Read the model definition and answer for the solid it produces. Units are mm, in the model's axes. A direction names the side the tool comes from. Give positions to 0.01 mm unless a question says otherwise; leave off trailing zeros. Order: outer loops, then holes, each group sorted by start corner. A loop starts at its lowest first (then second) coordinate and runs counter-clockwise, first axis right, second up. Notation, with made-up numbers: (20, 39) -> (49, 39) arc R32 cw to (49, 74) -> close; hole circle Ø8 at (-36, 7). An arc over 180 degrees is marked (long way). Answer as CSV lines item,"result". Start each with the question number.
1) Find section C-C (z = -7). Determine the outline of the cut face in (x, y).
2) Find section B-B (x = -14.5). Determine the outline of the cut face in (y, z), and give its area (3 significant figures).
3) Find section A-A (y = 10). Determine the outline of the cut face in (x, z), and give its area (3 significant figures).
4) Flat-ended cylindrical pins translate along their axes: pin 1 Ø0.9 at (y, z) = (1, -30.5) entering from -X; pin 2 Ø4 at (y, z) = (3.5, -33.5) entering from +X; pin 3 Ø5 at (x, y) = (-10, 8.5) entering from -Z (3 decimals); pin 4 Ø6 at (x, y) = (10, 12) entering from +Z. Find the tip coordinate at first contact, or state that the pin passes through.
5) Straight lines are drawn through the part: L1, parallel to Z at x = -1.5, y = 1; L2, parallel to Z at x = -31, y = 10; L3, parallel to Y at x = -14, z = -25. For each, find the intervals that lie inside material, in ascending order. Write a range as from..to.
6) For faces 5 (the face through (-28.911, 13.243, -14.867)), 6 (the face through (-16, 1, -2)), 7 (the face through (-5, 10, -24)), determine the directions among +Z, -Z, +X, -X, +Y, -Y from which every point of the face is accessible in a straight line to the end or side of a thin tool.
7) The mould has two halves that part along Z. Classify faces 1 (the face through (-3, 10, -45.888)), 2 (the face through (-15, 20, -15)), 3 (the face through (-22, 5, 14.112)), 4 (the face through (-28, 10, -33.888)): +Z half, -Z half, draft (parallel to the pull), parting line (faces both ways), or undercut.
8) Find section D-D (y = 3.5). Determine the outline of the cut face in (x, z).
```python
from build123d import *

# Parameters (mm, degrees)
F1_DEPTH = 20
F2_R     = 8.25
F3_DEPTH = 60.001
F5_D     = 6.8
F5_DEPTH = 20


with BuildPart() as f1:
    # F0 (on Front) → F1 (new body)
    with BuildSketch(Plane.XZ):
        Polygon((-36, -33.888159), (-36, -45.888159), (19, -45.888159), (19, -38.888159), (-5, -38.888159), (-5, -8.188159), (19, -8.188159), (19, -4.188159), (0, 14.111841), (-36, 14.111841), (-36, 2.111841), (-16, 2.111841), (-16, -5.888159), (-36, -5.888159), (-36, -25.888159), (-16, -25.888159), (-16, -33.888159), align=None)
    extrude(amount=-F1_DEPTH)

    # F2 (on face) → F3 (cut, through all)
    with BuildSketch(Plane.XY.offset(14.111841)):
        with Locations((-14.5, 10)):
            Circle(F2_R)
    extrude(amount=-F3_DEPTH, mode=Mode.SUBTRACT)

    # F5
    with Locations(Plane(origin=(-36, 0, 0), x_dir=(0, -1, 0), z_dir=(-1, 0, 0))):
        with Locations((-10, -15.888159)):
            Hole(F5_D / 2, depth=F5_DEPTH)


solid = f1.part
```
Findings below:
1,outline,"(-36, 0) -> (19, 0) -> (19, 20) -> (-36, 20) -> close; hole circle Ø16.5 at (-14.5, 10)"
2,outline,"(0, -45.89) -> (1.75, -45.89) -> (1.75, 14.11) -> (0, 14.11) -> close; (18.25, -45.89) -> (20, -45.89) -> (20, 14.11) -> (18.25, 14.11) -> close"
2,area,"210 mm²"
3,outline,"(-36, -45.89) -> (-22.75, -45.89) -> (-22.75, -33.89) -> (-36, -33.89) -> close; (-36, -25.89) -> (-22.75, -25.89) -> (-22.75, -19.29) -> (-36, -19.29) -> close; (-36, -12.49) -> (-22.75, -12.49) -> (-22.75, -5.89) -> (-36, -5.89) -> close; (-36, 2.11) -> (-22.75, 2.11) -> (-22.75, 14.11) -> (-36, 14.11) -> close; (-6.25, -45.89) -> (19, -45.89) -> (19, -38.89) -> (-5, -38.89) -> (-5, -8.19) -> (19, -8.19) -> (19, -4.19) -> (0, 14.11) -> (-6.25, 14.11) -> close"
3,area,"1,100 mm²"
4,pin 1,"x = -16"
4,pin 2,"x = -5"
4,pin 3,"through"
4,pin 4,"z = 7.37"
5,L1,"-45.89..-38.89, -8.19..14.11"
5,L2,"-45.89..-33.89, -25.89..-19.29, -12.49..-5.89, 2.11..14.11"
5,L3,"0..1.77, 18.23..20"
6,face 5,"-X"
6,face 6,"-X, +Y, -Y"
6,face 7,"+X, +Y, -Y"
7,face 1,"-Z half"
7,face 2,"draft"
7,face 3,"+Z half"
7,face 4,"undercut"
8,outline,"(-36, -45.89) -> (-19.58, -45.89) -> (-19.58, -33.89) -> (-36, -33.89) -> close; (-36, -25.89) -> (-19.58, -25.89) -> (-19.58, -5.89) -> (-36, -5.89) -> close; (-36, 2.11) -> (-19.58, 2.11) -> (-19.58, 14.11) -> (-36, 14.11) -> close; (-9.42, -45.89) -> (19, -45.89) -> (19, -38.89) -> (-5, -38.89) -> (-5, -8.19) -> (19, -8.19) -> (19, -4.19) -> (0, 14.11) -> (-9.42, 14.11) -> close"
